The listing builds one solid part. Answer for the finished solid, in the listing's coordinates (mm). Coordinates: 2 decimals unless noted, no trailing zeros. Write each loop counter-clockwise with the first axis right and the second up, starting at its lowest first coordinate (ties: lowest second). Pieces come first, ordered by that corner, then holes. Notation, with made-up numbers: M 59,17 L 88,17 A16 ccw 88,34 Z; hole C 15,64 d5. An arc over 180 degrees is marked long. Put each result on its own line as item: value. Start each with the question number.
```python
from build123d import *

# Parameters (mm, degrees)
SKETCH1_W          = 10
SKETCH1_H          = 85
CHAMFER1_SIZE      = 1
SKETCH2_R          = 0.5
CUT_EXTRUDE1_DEPTH = 3


with BuildPart() as part:
    # Sketch1 → Revolve1 (revolve)
    with BuildSketch(Plane(origin=(0, 0, 0), x_dir=(1, 0, 0), z_dir=(0, 1, 0)), mode=Mode.PRIVATE) as revolve1_sk:
        with Locations((5, 42.5)):
            Rectangle(SKETCH1_W, SKETCH1_H)
    revolve(revolve1_sk.sketch.rotate(Axis((0, 0, -85), (0, 0, 1)), 180), axis=Axis((0, 0, -85), (0, 0, 1)))

    # Chamfer1
    chamfer1_edges = [part.edges().sort_by_distance(p)[0] for p in [
        (10, 0, 0),
        (10, 0, -85),
    ]]
    chamfer(chamfer1_edges, length=CHAMFER1_SIZE)

    # Sketch2 → Cut-Extrude1 (cut)
    with BuildSketch(Plane(origin=(0, 0, -85), x_dir=(-1, 0, 0), z_dir=(0, 0, -1))):
        Circle(SKETCH2_R)
    extrude(amount=-CUT_EXTRUDE1_DEPTH, mode=Mode.SUBTRACT)


solid = part.part
```
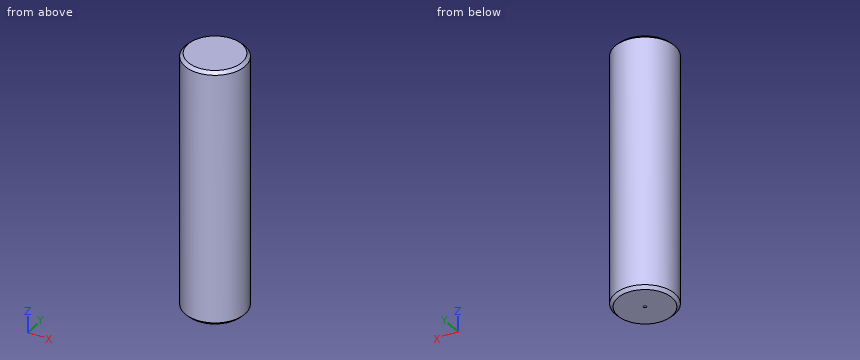
1) A cutting plane is placed at A-A on z = -79. Write down the section's boundary in (x, y).
2) Given pin 1 Ø6 at (x, z) = (-7, -36.5) entering from +Y; pin 2 Ø2 at (y, z) = (7, -25.5) entering from +X; pin 3 Ø4 at (y, z) = (-3.5, -70.5) entering from -X, each flat-ended and moving along its own axis, determine where each tip first touches the part or whether it passes through.
3) Straight lines are drawn through the part: probe 1 along Y at (x, z) = (0, -82.65); probe 2 along Y at (x, z) = (0, -46.5); probe 3 along X at (y, z) = (-7.25, -23). For each, find the intervals that lie inside material, in ascending order.
Answers follow:
1. outline: C 0,0 d20
2. pin 1: stops at y = 9.17
2. pin 2: stops at x = 8
2. pin 3: stops at x = -9.89
3. probe 1: y = -10 to -0.5, 0.5 to 10
3. probe 2: y = -10 to 10
3. probe 3: x = -6.89 to 6.89
